from build123d import *

# Parameters (mm, degrees)
SKETCH1_W           = 20
SKETCH1_H           = 25
BOSS_EXTRUDE1_DEPTH = 3
SKETCH3_W           = 23
SKETCH3_H           = 25
BOSS_EXTRUDE2_DEPTH = 3
SKETCH4_R           = 3
CUT_EXTRUDE1_DEPTH  = 27.930466019
SKETCH5_R           = 3
CUT_EXTRUDE2_DEPTH  = 33.94313282


with BuildPart() as part:
    # Sketch1 → Boss-Extrude1 (new body)
    with BuildSketch(Plane.XY):
        Rectangle(SKETCH1_W, SKETCH1_H)
    extrude(amount=BOSS_EXTRUDE1_DEPTH)

    # Sketch3 → Boss-Extrude2 (add)
    with BuildSketch(Plane(origin=(10, 0, 0), x_dir=(0, 0, -1), z_dir=(1, 0, 0))):
        with Locations((-11.5, 0)):
            Rectangle(SKETCH3_W, SKETCH3_H)
    extrude(amount=BOSS_EXTRUDE2_DEPTH)

    # Sketch4 → Cut-Extrude1 (cut, through all)
    with BuildSketch(Plane.XY.offset(3)):
        with Locations((0, 7)):
            Circle(SKETCH4_R)
        with Locations(Location((0, -7, 0), (0, 0, 180))):
            Circle(SKETCH4_R)
    extrude(amount=-CUT_EXTRUDE1_DEPTH, mode=Mode.SUBTRACT)

    # Sketch5 → Cut-Extrude2 (cut, through all)
    with BuildSketch(Plane.ZY.offset(-10)):
        with Locations((13, 7)):
            Circle(SKETCH5_R)
        with Locations(Location((13, -7, 0), (0, 0, 180))):
            Circle(SKETCH5_R)
    extrude(amount=-CUT_EXTRUDE2_DEPTH, mode=Mode.SUBTRACT)


solid = part.part
Check sheet for the modelled part. Datum: model origin and axes. Units: mm. A direction names the side the tool comes from. Give positions to 0.01 mm unless a question says otherwise; leave off trailing zeros. Write each loop counter-clockwise with the first axis right and the second up, starting at its lowest first coordinate (ties: lowest second). Pieces come first, ordered by that corner, then holes. Notation, with made-up numbers: (59.5, 22) -> (87.5, 22) arc R18 cw to (87.5, 34) -> close; hole circle Ø4 at (63.5, -22). An arc over 180 degrees is marked (long way). One line per item, written item: value. Start each with the question number.
Item 1: Tool access check on faces 4 (the cylindrical face through (11, 7, 10)), 5 (the flat face through (0, 0, 3)). Record the directions out of +Z, -Z, +X, -X, +Y, -Y that give a thin tool (end or side, any length) a straight path to the whole face; none if there is none.
Item 2: Material ranges on probe 1 along Y at (x, z) = (0, 0.9); probe 2 along Z at (x, y) = (11.9, -7); probe 3 along Z at (x, y) = (-2.5, -1.5), recorded low to high. Write a range as from..to.
Item 3: Gauge pin test, flat end, axial feed: pin 1 (8 mm diameter, centred on x = 0, y = -7, fed in from +Z). Record the tip position at first contact, or that the pin passes through.
Item 4: Section check B-B on y = 7. Record the cut outline in (x, z).
Item 5: Section check A-A on z = 13. Record the cut outline in (x, y).
Item 6: Section check C-C on x = 0. Record the cut outline in (y, z).
Item 7: Section check D-D on y = -2. Record the cut outline in (x, z).
Item 8: Draft check along X on faces 1 (the flat face through (1, 0, 0)), 2 (the flat face through (10, 0, 13)), 3 (the cylindrical face through (-3, 7, 2)). Enter one of: +X half, -X half, draft (parallel to the pull), parting line (faces both ways), or undercut.
Results list:
1. face 4: +X, -X
1. face 5: +Z, -X, +Y, -Y
2. probe 1: -12.5..-10, -4..4, 10..12.5
2. probe 2: 0..10, 16..23
2. probe 3: 0..3
3. pin 1: z = 3
4. outline: (-10, 0) -> (-3, 0) -> (-3, 3) -> (-10, 3) -> close; (3, 0) -> (13, 0) -> (13, 10) -> (10, 10) -> (10, 3) -> (3, 3) -> close; (10, 16) -> (13, 16) -> (13, 23) -> (10, 23) -> close
5. outline: (10, -12.5) -> (13, -12.5) -> (13, -10) -> (10, -10) -> close; (10, -4) -> (13, -4) -> (13, 4) -> (10, 4) -> close; (10, 10) -> (13, 10) -> (13, 12.5) -> (10, 12.5) -> close
6. outline: (-12.5, 0) -> (-10, 0) -> (-10, 3) -> (-12.5, 3) -> close; (-4, 0) -> (4, 0) -> (4, 3) -> (-4, 3) -> close; (10, 0) -> (12.5, 0) -> (12.5, 3) -> (10, 3) -> close
7. outline: (-10, 0) -> (13, 0) -> (13, 23) -> (10, 23) -> (10, 3) -> (-10, 3) -> close
8. face 1: draft
8. face 2: -X half
8. face 3: undercut
